Model file for the job. Use its own axes, mm. Face numbers are marked on the shaded views. Coordinates: 2 decimals unless noted, no trailing zeros. Write each loop counter-clockwise with the first axis right and the second up, starting at its lowest first coordinate (ties: lowest second). Pieces come first, ordered by that corner, then holes. Notation, with made-up numbers: M 12.25,29.5 L 63.25,29.5 A28 cw 63.25,67.5 Z; hole C -38,-34 d10. An arc over 180 degrees is marked long. One line per question, with ' | ' between items. Start each with the question number.
(1) Wall check: probe 1 along Z at (x, y) = (-0.95, 0); probe 2 along Z at (x, y) = (-7.75, 0). Give the ranges that are in metal, low to high.
(2) Cut at A-A (y = 0). Write the cut outline in (x, z), plus the area to 3 significant figures.
(3) Cut at D-D (y = -14). Write the cut outline in (x, z).
(4) Flat gauge pins, fed straight in: pin 1 Ø5 at (x, z) = (4.5, 12) entering from -Y; pin 2 Ø8 at (x, z) = (-4, -5.5) entering from -Y; pin 3 Ø1.5 at (x, z) = (3.5, 12.5) entering from -Y; pin 4 Ø16 at (y, z) = (0, 0) entering from -X. Where does each tip first touch, or does it go through?
(5) Two-plate mould, pull along Z, no slides. Class the marked faces 1, 2 and 3: +Z half, -Z half, draft (parallel to the pull), parting line (faces both ways), or undercut.
(6) Cut at C-C (x = 10.75). Write the cut outline in (y, z), plus the area to 3 significant figures.
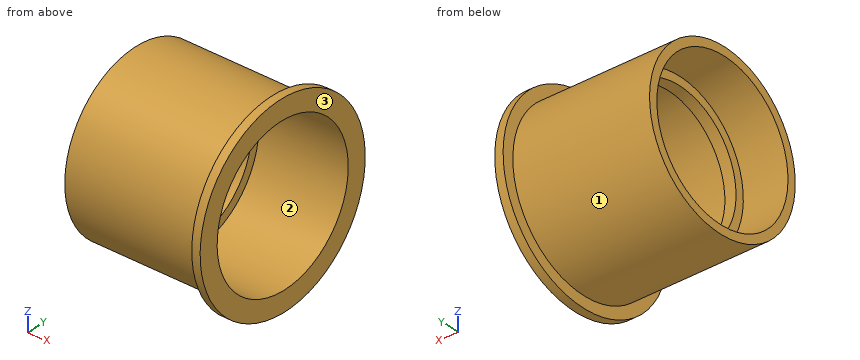
Autodesk Inventor part; units mm, degrees
ref_plane "YZ Plane" through (0, 0, 0) normal (1, 0, 0) x (0, 1, 0)
ref_plane "XZ Plane" through (0, 0, 0) normal (0, 1, 0) x (-1, 0, 0)
ref_plane "XY Plane" through (0, 0, 0) normal (0, 0, 1) x (1, 0, 0)
sketch "Sketch1" plane through (0, 0, 0) normal (0, 1, 0) x (-1, 0, 0)
  line L0 (0, 0) -> (10, 0)
  line L1 (2, -13.5) -> (10, -13.5)
  line L2 (2, -13.5) -> (2, -12)
  line L3 (2, -12) -> (0, -12)
  line L4 (10, -15) -> (10, -13.5)
  line L5 (0, -13.5) -> (-16, -13.5)
  line L6 (0, -13.5) -> (0, -12)
  line L7 (-16, -13.5) -> (-16, -17)
  line L8 (-16, -17) -> (-14.5, -17)
  line L9 (-14.5, -17) -> (-14.5, -15)
  line L10 (10, -15) -> (-14.5, -15)
  dimension "d0" = 1.5
  dimension "d4" = 1.5
  dimension "d5" = 10
  dimension "d7" = 24
  dimension "d8" = 27
  dimension "d11" = 16
  dimension "d12" = 27
  dimension "d13" = 1.5
  dimension "d14" = 34
  dimension "d16" = 2
revolve "Revolution1" add sketch "Sketch1" angle 360 about axis through (0, 0, 0) along (-1, 0, 0)
thread "Thread1"
properties part number "030" material "Aluminum 6061"
Filled in:
1) probe 1: -15 to -12, 12 to 15 | probe 2: -15 to -13.5, 13.5 to 15
2) outline: M -10,-15 L 14.5,-15 L 14.5,-17 L 16,-17 L 16,-13.5 L 0,-13.5 L 0,-12 L -2,-12 L -2,-13.5 L -10,-13.5 Z; M -10,13.5 L -2,13.5 L -2,12 L 0,12 L 0,13.5 L 16,13.5 L 16,17 L 14.5,17 L 14.5,15 L -10,15 Z | area: 90.0 mm²
3) outline: M -10,-5.39 L 14.5,-5.39 L 14.5,-9.64 L 16,-9.64 L 16,9.64 L 14.5,9.64 L 14.5,5.39 L -10,5.39 Z
4) pin 1: y = -11.61 | pin 2: y = -14.92 | pin 3: y = -9.32 | pin 4: through
5) face 1: parting line | face 2: undercut | face 3: draft
6) outline: C 0,0 d30; hole C 0,0 d27 | area: 134 mm²
